```python
from build123d import *

# Parameters (mm, degrees)
FILLET1_R          = 0.1
CUT_EXTRUDE1_DEPTH = 1


with BuildPart() as part:
    # Sketch1 → Revolve1 (revolve)
    with BuildSketch(Plane.XY, mode=Mode.PRIVATE) as revolve1_sk:
        Polygon((0, 0), (-3, 0), (-3, -1.5), (-1.25, -1.5), (-1.25, -16.5), (0, -16.5), align=None)
    revolve(revolve1_sk.sketch.rotate(Axis((0, 14.912855268, 0), (0, -1, 0)), 270), axis=Axis((0, 14.912855268, 0), (0, -1, 0)))

    # Fillet1
    fillet1_edges = [part.edges().sort_by_distance(p)[0] for p in [
        (0, -16.5, -1.25),
        (0, -1.5, -3),
        (0, 0, -3),
    ]]
    fillet(fillet1_edges, radius=FILLET1_R)

    # Sketch2 → Cut-Extrude1 (cut)
    with BuildSketch(Plane(origin=(0, 0, 0), x_dir=(1, 0, 0), z_dir=(0, 1, 0))):
        with BuildLine():
            Line((-2.214158983, -0.4), (-0.6, -0.4))
            ThreePointArc((-0.6, -0.4), (-0.458578644, -0.458578644), (-0.4, -0.6))
            Line((-0.4, -0.6), (-0.4, -2.214158983))
            ThreePointArc((-0.4, -2.214158983), (0, -2.25), (0.4, -2.214158983))
            Line((0.4, -2.214158983), (0.4, -0.6))
            ThreePointArc((0.4, -0.6), (0.458578644, -0.458578644), (0.6, -0.4))
            Line((0.6, -0.4), (2.214158983, -0.4))
            ThreePointArc((2.214158983, -0.4), (2.25, 0), (2.214158983, 0.4))
            Line((2.214158983, 0.4), (0.6, 0.4))
            ThreePointArc((0.6, 0.4), (0.458578644, 0.458578644), (0.4, 0.6))
            Line((0.4, 0.6), (0.4, 2.214158983))
            ThreePointArc((0.4, 2.214158983), (0, 2.25), (-0.4, 2.214158983))
            Line((-0.4, 2.214158983), (-0.4, 0.6))
            ThreePointArc((-0.4, 0.6), (-0.458578644, 0.458578644), (-0.6, 0.4))
            Line((-0.6, 0.4), (-2.214158983, 0.4))
            ThreePointArc((-2.214158983, 0.4), (-2.25, 0), (-2.214158983, -0.4))
        make_face()
    extrude(amount=-CUT_EXTRUDE1_DEPTH, mode=Mode.SUBTRACT)


solid = part.part
```
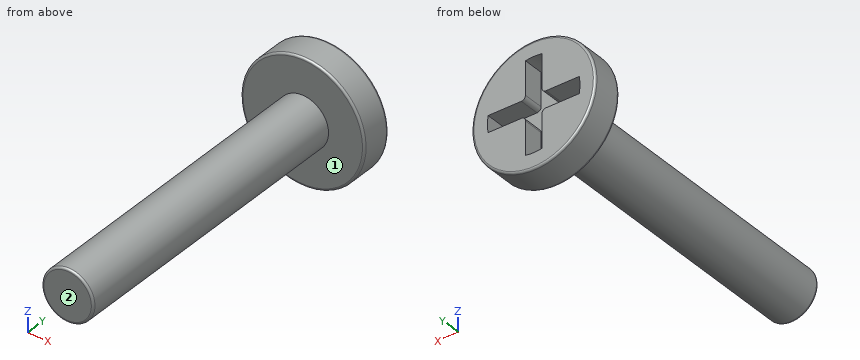
Geometry check sheet. Reference: the model listing, model coordinates, mm. Face numbers are marked on the shaded views. A direction names the side the tool comes from. Coordinates: 2 decimals unless noted, no trailing zeros. Order: outer loops, then holes, each group sorted by start corner. A loop starts at its lowest first (then second) coordinate and runs counter-clockwise, first axis right, second up. Notation, with made-up numbers: M 27.5,-39 L 40.5,-39 A11 ccw 40.5,-30 Z; hole C -12.5,-26 d10. An arc over 180 degrees is marked long. Answer as a JSON object with one key per item and string values.
Q1. Depth check by flat-ended pin: pin 1 Ø0.8 at (y, z) = (-0.5, -1.5) entering from -X; pin 2 Ø1.5 at (y, z) = (-10, 0) entering from -X; pin 3 Ø0.5 at (y, z) = (-0.5, 1.5) entering from -X. Enter the tip coordinate at first touch or a pass-through.
Results are:
{"pin 1": "stops at x = -2.79", "pin 2": "stops at x = -1.25", "pin 3": "stops at x = -2.73"}
Q2. Scan lines: line 1 (X direction, y = -11.25, z = 0.5); line 2 (Y direction, x = 2, z = -1). Record each from-to range of solid material in increasing order.
Results are:
{"line 1": "x = -1.15 to 1.15", "line 2": "y = -1.5 to 0"}
Q3. Cross-section at A-A on x = 0. Record the cut outline in (y, z), and give its area (3 significant figures).
Results are:
{"outline": "M -16.5,-1.15 A0.1 ccw -16.4,-1.25 L -1.5,-1.25 L -1.5,-2.9 A0.1 ccw -1.4,-3 L -0.1,-3 A0.1 ccw 0,-2.9 L 0,-2.25 L -1,-2.25 L -1,2.25 L 0,2.25 L 0,2.9 A0.1 ccw -0.1,3 L -1.4,3 A0.1 ccw -1.5,2.9 L -1.5,1.25 L -16.4,1.25 A0.1 ccw -16.5,1.15 Z", "area": "42.0 mm²"}
Q4. Tool access check on the marked faces 1 and 2. Record the directions out of +Z, -Z, +X, -X, +Y, -Y that give a thin tool (end or side, any length) a straight path to the whole face; none if there is none.
Results are:
{"face 1": "-Y", "face 2": "+Z, -Z, +X, -X, -Y"}
Q5. Cross-section at C-C on y = -4.5. Record the cut outline in (x, z), and give its area (3 significant figures).
Results are:
{"outline": "C 0,0 d2.5", "area": "4.91 mm²"}
Q6. Cross-section at B-B on z = 0. Record the cut outline in (x, y), and give its area (3 significant figures).
Results are:
{"outline": "M -3,-1.4 A0.1 ccw -2.9,-1.5 L -1.25,-1.5 L -1.25,-16.4 A0.1 ccw -1.15,-16.5 L 1.15,-16.5 A0.1 ccw 1.25,-16.4 L 1.25,-1.5 L 2.9,-1.5 A0.1 ccw 3,-1.4 L 3,-0.1 A0.1 ccw 2.9,0 L 2.25,0 L 2.25,-1 L -2.25,-1 L -2.25,0 L -2.9,0 A0.1 ccw -3,-0.1 Z", "area": "42.0 mm²"}
